```python
from build123d import *

# Parameters (mm, degrees)
IZIM1_W                     = 170
IZIM1_H                     = 104
Y_KSEKLIK_EKSTR_ZYON1_DEPTH = 4
Y_KSEKLIK_EKSTR_ZYON2_DEPTH = 55
IZIM3_R                     = 2.55
KES_EKSTR_ZYON1_DEPTH       = 12
KES_EKSTR_ZYON2_DEPTH       = 7
IZIM5_R                     = 2.1
KES_EKSTR_ZYON3_DEPTH       = 5
IZIM7_R                     = 4.4
KES_EKSTR_ZYON5_DEPTH       = 3.5


with BuildPart() as part:
    # Çizim1 → Yükseklik-Ekstrüzyon1 (new, symmetric)
    with BuildSketch(Plane.XY):
        Rectangle(IZIM1_W, IZIM1_H)
    extrude(amount=Y_KSEKLIK_EKSTR_ZYON1_DEPTH, both=True)

    # Çizim2 → Yükseklik-Ekstrüzyon2 (add, symmetric)
    with BuildSketch(Plane(origin=(0, 0, 0), x_dir=(1, 0, 0), z_dir=(0, 1, 0))):
        with BuildLine():
            Line((-74.9, 1.45), (-45.1, 1.45))
            ThreePointArc((-45.1, 1.45), (-43.65, 0), (-45.1, -1.45))
            Line((-45.1, -1.45), (-74.9, -1.45))
            ThreePointArc((-74.9, -1.45), (-76.35, 0), (-74.9, 1.45))
        make_face()
        with BuildLine():
            Line((-14.9, 1.45), (14.9, 1.45))
            ThreePointArc((14.9, 1.45), (16.35, 0), (14.9, -1.45))
            Line((14.9, -1.45), (-14.9, -1.45))
            ThreePointArc((-14.9, -1.45), (-16.35, 0), (-14.9, 1.45))
        make_face()
        with BuildLine():
            Line((45.1, 1.45), (74.9, 1.45))
            ThreePointArc((74.9, 1.45), (76.35, 0), (74.9, -1.45))
            Line((74.9, -1.45), (45.1, -1.45))
            ThreePointArc((45.1, -1.45), (43.65, 0), (45.1, 1.45))
        make_face()
    extrude(amount=Y_KSEKLIK_EKSTR_ZYON2_DEPTH, both=True)

    # Çizim3 → Kes-Ekstrüzyon1 (cut)
    with BuildSketch(Plane(origin=(0, 52, 0), x_dir=(1, 0, 0), z_dir=(0, 1, 0))):
        with Locations(Location((-30, 0, 0), (0, 0, 270))):
            Circle(IZIM3_R)
        with Locations(Location((30, 0, 0), (0, 0, 270))):
            Circle(IZIM3_R)
    kes_ekstr_zyon1 = extrude(amount=-KES_EKSTR_ZYON1_DEPTH, mode=Mode.SUBTRACT)

    # Aynalama1: Kes-Ekstrüzyon1 across plane
    add(kes_ekstr_zyon1.mirror(Plane.ZX), mode=Mode.SUBTRACT)

    # Çizim4 → Kes-Ekstrüzyon2 (cut)
    with BuildSketch(Plane.ZY.offset(85)):
        with BuildLine():
            Line((-1.65, -45.1), (-1.65, -14.9))
            ThreePointArc((-1.65, -14.9), (0, -13.25), (1.65, -14.9))
            Line((1.65, -14.9), (1.65, -45.1))
            ThreePointArc((1.65, -45.1), (0, -46.75), (-1.65, -45.1))
        make_face()
        with BuildLine():
            Line((-1.65, 14.9), (-1.65, 45.1))
            ThreePointArc((-1.65, 45.1), (0, 46.75), (1.65, 45.1))
            Line((1.65, 45.1), (1.65, 14.9))
            ThreePointArc((1.65, 14.9), (0, 13.25), (-1.65, 14.9))
        make_face()
    kes_ekstr_zyon2 = extrude(amount=-KES_EKSTR_ZYON2_DEPTH, mode=Mode.SUBTRACT)

    # Çizim5 → Kes-Ekstrüzyon3 (cut, symmetric)
    with BuildSketch(Plane.XY):
        with Locations((-76, 0)):
            Circle(IZIM5_R)
    kes_ekstr_zyon3 = extrude(amount=KES_EKSTR_ZYON3_DEPTH, both=True, mode=Mode.SUBTRACT)

    # Çizim7 → Kes-Ekstrüzyon5 (cut)
    with BuildSketch(Plane(origin=(0, 0, -4), x_dir=(-1, 0, 0), z_dir=(0, 0, -1))):
        with Locations((76, 0)):
            Circle(IZIM7_R)
    kes_ekstr_zyon5 = extrude(amount=-KES_EKSTR_ZYON5_DEPTH, mode=Mode.SUBTRACT)

    # Aynalama2: Kes-Ekstrüzyon2, Kes-Ekstrüzyon3, Kes-Ekstrüzyon5 across plane
    add(kes_ekstr_zyon2.mirror(Plane(origin=(0, 0, 0), x_dir=(0, 0, 1), z_dir=(1, 0, 0))), mode=Mode.SUBTRACT)
    add(kes_ekstr_zyon3.mirror(Plane(origin=(0, 0, 0), x_dir=(0, 0, 1), z_dir=(1, 0, 0))), mode=Mode.SUBTRACT)
    add(kes_ekstr_zyon5.mirror(Plane(origin=(0, 0, 0), x_dir=(0, 0, 1), z_dir=(1, 0, 0))), mode=Mode.SUBTRACT)


solid = part.part
```
Here's how the part is built. I have some questions about the finished solid (model axes, mm). A direction names the side the tool comes from. Coordinates: 2 decimals unless noted, no trailing zeros. Order: outer loops, then holes, each group sorted by start corner. A loop starts at its lowest first (then second) coordinate and runs counter-clockwise, first axis right, second up. Notation, with made-up numbers: (43, -35) - (90, -35) arc R27 ccw to (90, -12) - close; hole circle Ø10 at (-36.75, 57). An arc over 180 degrees is marked (long way). One line per question, with ' | ' between items.
(1) Suppose I cut it at B-B on y = -37. List the corners of the cut face in (x, z) for me, and give its area (3 significant figures).
Report:
outline: (-85, -4) - (85, -4) - (85, -1.65) - (78, -1.65) - (78, 1.65) - (85, 1.65) - (85, 4) - (-85, 4) - (-85, 1.65) - (-78, 1.65) - (-78, -1.65) - (-85, -1.65) - close | area: 1,310 mm2
(2) For faces 5 (the flat face through (78, -30, 0)), 6 (the cylindrical face through (-81.55, -13.25, -0.04)), 7 (the flat face through (30, -40, 0)), which set-ups out of +Z, -Z, +X, -X, +Y, -Y let a thin tool reach every point of the face, with its end or its side?
Report:
face 5: +X | face 6: -X | face 7: -Y
(3) Will these pins go through, and if not, where does the flat tip stop? pin 1 (0.9 mm diameter, centred on x = -60.5, y = -53.5, fed in from +Z); pin 2 (1.5 mm diameter, centred on x = -30.5, z = 1, fed in from -Y); pin 3 (4.5 mm diameter, centred on x = 75.5, y = -1.5, fed in from -Z).
Report:
pin 1: stops at z = 1.45 | pin 2: stops at y = -40 | pin 3: stops at z = -0.5
(4) If I drill on L1, parallel to X at y = -47, z = 0; L2, parallel to X at y = -45.25, z = 0; L3, parallel to Y at x = -76, z = 0.45, over which ranges is the centre line in solid material (lowest first)?
Report:
L1: x = -85 to -32.55, -27.45 to 27.45, 32.55 to 85 | L2: x = -78 to -32.55, -27.45 to 27.45, 32.55 to 78 | L3: y = -55 to -2.1, 2.1 to 55
(5) If we mould it in two halves opening along X, with no side actions, what happens to faces 1 (the cylindrical face through (32.53, 46.08, -0.33)), 2 (the flat face through (85, -1, 0)), 3 (the flat face through (-78, -30, 0)), 4 (the flat face through (-82, 30, -1.65))? For each: pulls with the +X half, pulls with the -X half, needs draft (parallel to the pull), parting line crosses it, or undercut.
Report:
face 1: undercut | face 2: pulls with the +X half | face 3: pulls with the -X half | face 4: needs draft
(6) Suppose I cut it at A-A on x = 57. List the corners of the cut face in (y, z) for me, and give its area (3 significant figures).
Report:
outline: (-55, -1.45) - (-52, -1.45) - (-52, -4) - (52, -4) - (52, -1.45) - (55, -1.45) - (55, 1.45) - (52, 1.45) - (52, 4) - (-52, 4) - (-52, 1.45) - (-55, 1.45) - close | area: 849 mm2
